Read the model definition and answer for the solid it produces. Units are mm, in the model's axes. A direction names the side the tool comes from. Coordinates: 2 decimals unless noted, no trailing zeros. Order: outer loops, then holes, each group sorted by start corner. A loop starts at its lowest first (then second) coordinate and runs counter-clockwise, first axis right, second up. Notation, with made-up numbers: (-21, 24) -> (-4, 24) arc R25 cw to (-4, 63) -> close; hole circle Ø6 at (11.25, 17). An arc over 180 degrees is marked (long way). Answer as a JSON object with one key per item and string values. Group by question number.
1) Given pin 1 (12 mm diameter, centred on x = 9.5, y = 62.5, fed in from +Z); pin 2 (2 mm diameter, centred on y = 14, z = -41, fed in from -X); pin 3 (2 mm diameter, centred on x = 1, z = -13.5, fed in from +Y), each flat-ended and moving along its own axis, determine where each tip first touches the part or whether it passes through.
2) Section D-D on x = 10 is taken. Determine the outline of the cut face in (y, z), and give its area (3 significant figures).
3) Section B-B on z = 0 is taken. Determine the outline of the cut face in (x, y).
4) Section A-A on y = 0 is taken. Determine the outline of the cut face in (x, z), and give its area (3 significant figures).
5) A tool of negligible diameter and unlimited length cuts with its end or side. For faces 1 (the cylindrical face through (-7.535, -39.923, 20.765)), 2 (the cylindrical face through (-2.54, -9.76, -2.17)), 3 (the flat face through (0, 1, -17)), from which of +Z, -Z, +X, -X, +Y, -Y can it reach the whole face along a straight path? Write none if from no direction.
6) Consider L1, parallel to X at y = 38, z = 29; L2, parallel to Z at x = 25.5, y = 10; L3, parallel to Z at x = -1.5, y = -26.5. Determine where each line is inside the solid, lowest interval first.
7) Section C-C on x = -3 is taken. Determine the outline of the cut face in (y, z).
8) Determine the mould class of faces 4 (the cylindrical face through (12.255, -11.195, 85.268)), 5 (the cylindrical face through (-2.535, -29.842, -17.257)), 6 (the flat face through (-10, 35, -35)) for opening direction Y: released by +Y, released by -Y, zero draft, split by the parting line, or undercut.
from build123d import *

# Parameters (mm, degrees)
FILLET1_R          = 5
SKETCH2_R          = 45
CUT_EXTRUDE1_DEPTH = 5
SKETCH3_R          = 10
CUT_EXTRUDE2_DEPTH = 41
CUT_EXTRUDE3_REACH = 37
SKETCH4_R          = 4


with BuildPart() as part:
    # Sketch1 → Revolve1 (revolve)
    with BuildSketch(Plane.XY):
        Polygon((0, 0), (0, 81), (30, 81), (30, 86), (-10, 86), (-10, 0), align=None)
    revolve(axis=Axis((-10, 0, 0), (1, 0, 0)))

    # Fillet1
    fillet1_edges = [part.edges().sort_by_distance(p)[0] for p in [
        (-10, -86, 0),
    ]]
    fillet(fillet1_edges, radius=FILLET1_R)

    # Sketch2 → Cut-Extrude1 (cut)
    with BuildSketch(Plane.ZY.offset(10)):
        Circle(SKETCH2_R)
    extrude(amount=-CUT_EXTRUDE1_DEPTH, mode=Mode.SUBTRACT)

    # Sketch3 → Cut-Extrude2 (cut, through all)
    with BuildSketch(Plane.ZY.offset(10)):
        Circle(SKETCH3_R)
    extrude(amount=-CUT_EXTRUDE2_DEPTH, mode=Mode.SUBTRACT)

    # Sketch4 → Cut-Extrude3 (cut, up to next)
    with BuildSketch(Plane.ZY.offset(5), mode=Mode.PRIVATE) as cut_extrude3_sk1:
        with Locations((0, 32.5)):
            Circle(SKETCH4_R)
    cut_extrude3_tool1 = extrude(cut_extrude3_sk1.sketch, amount=-CUT_EXTRUDE3_REACH, mode=Mode.PRIVATE) & part.part
    add(cut_extrude3_tool1.solids().sort_by_distance((-5, 32.5, 0))[0], mode=Mode.SUBTRACT)
    # Sketch4 → Cut-Extrude3 (cut, up to next)
    with BuildSketch(Plane.ZY.offset(5), mode=Mode.PRIVATE) as cut_extrude3_sk2:
        with Locations((30.90933678, 10.043052317)):
            Circle(SKETCH4_R)
    cut_extrude3_tool2 = extrude(cut_extrude3_sk2.sketch, amount=-CUT_EXTRUDE3_REACH, mode=Mode.PRIVATE) & part.part
    add(cut_extrude3_tool2.solids().sort_by_distance((-5, 10.043052, 30.909337))[0], mode=Mode.SUBTRACT)
    # Sketch4 → Cut-Extrude3 (cut, up to next)
    with BuildSketch(Plane.ZY.offset(5), mode=Mode.PRIVATE) as cut_extrude3_sk3:
        with Locations((19.1030207, -26.293052317)):
            Circle(SKETCH4_R)
    cut_extrude3_tool3 = extrude(cut_extrude3_sk3.sketch, amount=-CUT_EXTRUDE3_REACH, mode=Mode.PRIVATE) & part.part
    add(cut_extrude3_tool3.solids().sort_by_distance((-5, -26.293052, 19.103021))[0], mode=Mode.SUBTRACT)
    # Sketch4 → Cut-Extrude3 (cut, up to next)
    with BuildSketch(Plane.ZY.offset(5), mode=Mode.PRIVATE) as cut_extrude3_sk4:
        with Locations((-19.1030207, -26.293052317)):
            Circle(SKETCH4_R)
    cut_extrude3_tool4 = extrude(cut_extrude3_sk4.sketch, amount=-CUT_EXTRUDE3_REACH, mode=Mode.PRIVATE) & part.part
    add(cut_extrude3_tool4.solids().sort_by_distance((-5, -26.293052, -19.103021))[0], mode=Mode.SUBTRACT)
    # Sketch4 → Cut-Extrude3 (cut, up to next)
    with BuildSketch(Plane.ZY.offset(5), mode=Mode.PRIVATE) as cut_extrude3_sk5:
        with Locations((-30.90933678, 10.043052317)):
            Circle(SKETCH4_R)
    cut_extrude3_tool5 = extrude(cut_extrude3_sk5.sketch, amount=-CUT_EXTRUDE3_REACH, mode=Mode.PRIVATE) & part.part
    add(cut_extrude3_tool5.solids().sort_by_distance((-5, 10.043052, -30.909337))[0], mode=Mode.SUBTRACT)


solid = part.part
Worked answers:
{
 "1": {"pin 1": "stops at z = 64.84", "pin 2": "stops at x = -5", "pin 3": "stops at y = 85.09"},
 "2": {"outline": "circle Ø172 at (0, 0); hole circle Ø162 at (0, 0)", "area": "2,620 mm²"},
 "3": {"outline": "(-10, -81) arc R5 ccw to (-5, -86) -> (30, -86) -> (30, -81) -> (0, -81) -> (0, -10) -> (-5, -10) -> (-5, -45) -> (-10, -45) -> close; (-10, 45) -> (-5, 45) -> (-5, 36.5) -> (0, 36.5) -> (0, 81) -> (30, 81) -> (30, 86) -> (-5, 86) arc R5 ccw to (-10, 81) -> close; (-5, 10) -> (0, 10) -> (0, 28.5) -> (-5, 28.5) -> close"},
 "4": {"outline": "(-10, -81) arc R5 ccw to (-5, -86) -> (30, -86) -> (30, -81) -> (0, -81) -> (0, -10) -> (-5, -10) -> (-5, -45) -> (-10, -45) -> close; (-10, 45) -> (-5, 45) -> (-5, 10) -> (0, 10) -> (0, 81) -> (30, 81) -> (30, 86) -> (-5, 86) arc R5 ccw to (-10, 81) -> close", "area": "1,460 mm²"},
 "5": {"face 1": "-X", "face 2": "+X, -X", "face 3": "+X"},
 "6": {"L1": "x = -10 to 0", "L2": "z = -85.42 to -80.38, 80.38 to 85.42", "L3": "z = -81.82 to -23.1, -15.11 to 15.11, 23.1 to 81.82"},
 "7": {"outline": "circle Ø172 at (0, 0); hole circle Ø8 at (-26.29, -19.1); hole circle Ø8 at (-26.29, 19.1); hole circle Ø20 at (0, 0); hole circle Ø8 at (10.04, -30.91); hole circle Ø8 at (10.04, 30.91); hole circle Ø8 at (32.5, 0)"},
 "8": {"face 4": "split by the parting line", "face 5": "undercut", "face 6": "zero draft"}
}
